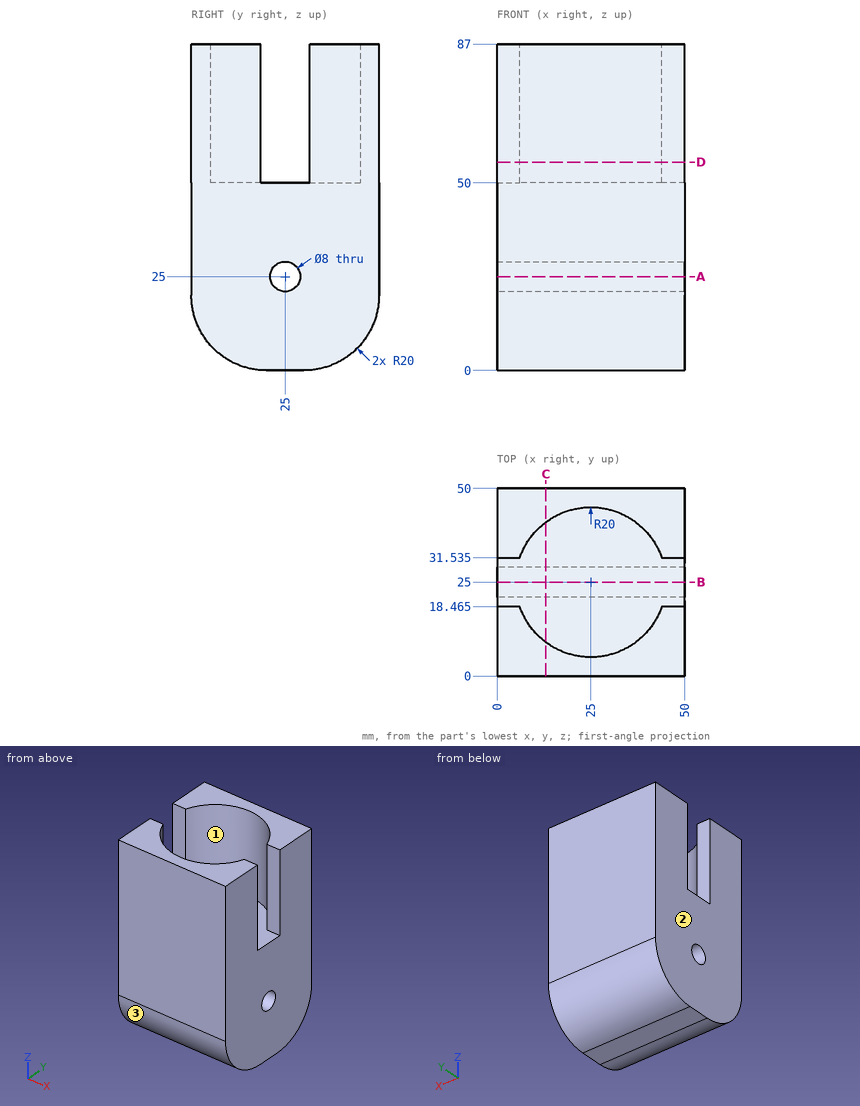
Print and shaded views of the part. All mm, measured from the part's lowest x, y and z. Coordinates: 2 decimals unless noted, no trailing zeros. Order: outer loops, then holes, each group sorted by start corner. A loop starts at its lowest first (then second) coordinate and runs counter-clockwise, first axis right, second up.
Item 1: Saw through at A-A on z = 25. List the corners of the cut face in (x, y), then the cut area to 3 significant figures.
Filled in:
outline: (0, 0) - (50, 0) - (50, 21) - (0, 21) - close; (0, 29) - (50, 29) - (50, 50) - (0, 50) - close
area: 2,100 mm2
Item 2: Saw through at D-D on z = 55.5. List the corners of the cut face in (x, y) (3 decimals), then the cut area to 3 significant figures.
Filled in:
outline: (0, 0) - (50, 0) - (50, 18.465) - (43.902, 18.465) arc R20 cw to (6.098, 18.465) - (0, 18.465) - close; (0, 31.535) - (6.098, 31.535) arc R20 cw to (43.902, 31.535) - (50, 31.535) - (50, 50) - (0, 50) - close
area: 1,100 mm2
Item 3: Saw through at C-C on x = 13. List the corners of the cut face in (y, z), then the cut area to 3 significant figures.
Filled in:
outline: (0, 20) arc R20 ccw to (20, 0) - (30, 0) arc R20 ccw to (50, 20) - (50, 87) - (41, 87) - (41, 50) - (9, 50) - (9, 87) - (0, 87) - close; hole circle Ø8 at (25, 25)
area: 2,940 mm2
Item 4: Drill centre lines: L1, parallel to Y at x = 20.5, z = 25; L2, parallel to Y at x = 3, z = 68.5 (3 decimals); L3, parallel to Z at x = 35, y = 19.5. Where is each one in solid material? Low to high.
Filled in:
L1: y = 0 to 21, 29 to 50
L2: y = 0 to 18.465, 31.535 to 50
L3: z = 0.01 to 50
Item 5: Drop flat-ended pins along their axis: pin 1 Ø3 at (y, z) = (16.5, 68.5) entering from -X; pin 2 Ø3 at (x, y) = (38.5, 27.5) entering from +Z; pin 3 Ø2 at (x, y) = (9, 5.5) entering from -Z; pin 4 Ø6 at (x, y) = (6.5, 39.5) entering from -Z. Give the stop position or say it passes through.
Filled in:
pin 1: stops at x = 0
pin 2: stops at z = 50
pin 3: stops at z = 5.24
pin 4: stops at z = 1.09
Item 6: Mould opens along X. For the marked faces 1, 2 and 3 say: released by +X, released by -X, zero draft, split by the parting line, or undercut.
Filled in:
face 1: undercut
face 2: released by -X
face 3: zero draft
